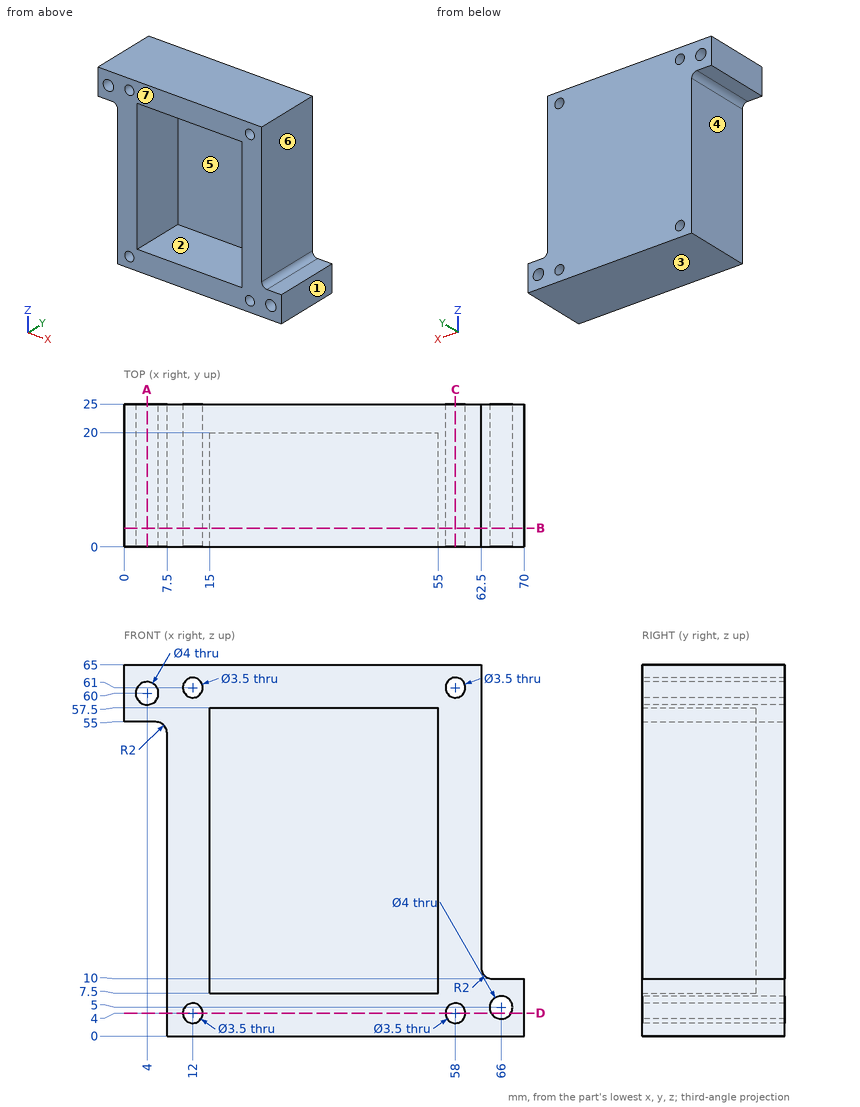
Could you check a few things on this drawing? It's one solid part, dimensions in mm from its lowest x, y, z. A direction names the side the tool comes from. Round coordinates to 2 decimals unless told otherwise and drop trailing zeros. Loops run counter-clockwise (first coordinate to the right, second up) from the corner with the lowest first, then second, coordinate; pieces in that order, holes last. Notation, with made-up numbers: (85, 78.25) -> (141, 78.25) arc R22 ccw to (141, 88.25) -> close; hole circle Ø3 at (11, 15). An arc over 180 degrees is marked (long way). One line per item, written item: value. Start each with the question number.
1. If we section it at A-A, the plane x = 4: Write out the boundary of the cut face in (y, z).
2. If we section it at C-C, the plane x = 58: Write out the boundary of the cut face in (y, z).
3. For pin 1 (1.5 mm diameter, centred on x = 34, z = 31.5, fed in from -Y); pin 2 (4.5 mm diameter, centred on x = 4, y = 12.5, fed in from -Z); pin 3 (6 mm diameter, centred on x = 66, y = 11, fed in from +Z), each with a flat end and sliding along its axis, tell me the tip position at first contact or that it passes through.
4. If we mould it in two halves opening along X, with no side actions, what happens to the marked faces 1, 2 and 3? For each: pulls with the +X half, pulls with the -X half, needs draft (parallel to the pull), parting line crosses it, or undercut.
5. For the marked faces 4, 5, 6 and 7, which set-ups out of +Z, -Z, +X, -X, +Y, -Y let a thin tool reach every point of the face, with its end or its side?
6. If we section it at D-D, the plane z = 4: Write out the boundary of the cut face in (x, y).
7. If we section it at B-B, the plane y = 3.25: Write out the boundary of the cut face in (x, z).
8. If I drill on probe 1 along Z at (x, y) = (12, 8); probe 2 along Z at (x, y) = (4, 11); probe 3 along Z at (x, y) = (39, 3.75), over which ranges is the centre line in solid material (lowest first)?
Calculated:
1. outline: (0, 55) -> (25, 55) -> (25, 58) -> (0, 58) -> close; (0, 62) -> (25, 62) -> (25, 65) -> (0, 65) -> close
2. outline: (0, 0) -> (25, 0) -> (25, 2.25) -> (0, 2.25) -> close; (0, 5.75) -> (25, 5.75) -> (25, 59.25) -> (0, 59.25) -> close; (0, 62.75) -> (25, 62.75) -> (25, 65) -> (0, 65) -> close
3. pin 1: stops at y = 20
3. pin 2: stops at z = 54.85
3. pin 3: stops at z = 10.68
4. face 1: pulls with the +X half
4. face 2: undercut
4. face 3: needs draft
5. face 4: -Z, -X, +Y, -Y
5. face 5: -Y
5. face 6: +Z, +X, +Y, -Y
5. face 7: +Z, -Z, +X, -X, -Y
6. outline: (7.5, 0) -> (10.25, 0) -> (10.25, 25) -> (7.5, 25) -> close; (13.75, 0) -> (56.25, 0) -> (56.25, 25) -> (13.75, 25) -> close; (59.75, 0) -> (64.27, 0) -> (64.27, 25) -> (59.75, 25) -> close; (67.73, 0) -> (70, 0) -> (70, 25) -> (67.73, 25) -> close
7. outline: (0, 55) -> (5.5, 55) arc R2 cw to (7.5, 53) -> (7.5, 0) -> (70, 0) -> (70, 10) -> (64.5, 10) arc R2 cw to (62.5, 12) -> (62.5, 65) -> (0, 65) -> close; hole circle Ø4 at (4, 60); hole circle Ø3.5 at (12, 4); hole circle Ø3.5 at (12, 61); hole (15, 7.5) -> (55, 7.5) -> (55, 57.5) -> (15, 57.5) -> close; hole circle Ø3.5 at (58, 4); hole circle Ø3.5 at (58, 61); hole circle Ø4 at (66, 5)
8. probe 1: z = 0 to 2.25, 5.75 to 59.25, 62.75 to 65
8. probe 2: z = 55 to 58, 62 to 65
8. probe 3: z = 0 to 7.5, 57.5 to 65
